```python
from build123d import *

# Parameters (mm, degrees)
SKETCH1_R           = 50
SKETCH1_W           = 15
SKETCH1_H           = 4
SKETCH1_W_2         = 4
SKETCH1_H_2         = 15
BOSS_EXTRUDE1_DEPTH = 5


with BuildPart() as part:
    # Sketch1 → Boss-Extrude1 (new body)
    with BuildSketch(Plane.XY):
        Circle(SKETCH1_R)
        with BuildLine():
            Line((-5, 14.142135624), (-5, 18.3))
            Line((-5, 18.3), (5, 18.3))
            Line((5, 18.3), (5, 14.142135624))
            ThreePointArc((5, 14.142135624), (0, -15), (-5, 14.142135624))
        make_face(mode=Mode.SUBTRACT)
        with Locations((-35, 0)):
            Rectangle(SKETCH1_W, SKETCH1_H, mode=Mode.SUBTRACT)
        Polygon((-38.499513267, 18.111804941), (-24.641320279, 12.371553455), (-26.172054009, 8.676035325), (-40.030246996, 14.41628681), align=None, mode=Mode.SUBTRACT)
        Polygon((-28.637824638, 31.466251763), (-18.03122292, 20.859650045), (-20.859650045, 18.03122292), (-31.466251763, 28.637824638), align=None, mode=Mode.SUBTRACT)
        Polygon((-14.41628681, 40.030246996), (-8.676035325, 26.172054009), (-12.371553455, 24.641320279), (-18.111804941, 38.499513267), align=None, mode=Mode.SUBTRACT)
        with Locations((0, 35)):
            Rectangle(SKETCH1_W_2, SKETCH1_H_2, mode=Mode.SUBTRACT)
        Polygon((18.111804941, 38.499513267), (12.371553455, 24.641320279), (8.676035325, 26.172054009), (14.41628681, 40.030246996), align=None, mode=Mode.SUBTRACT)
        Polygon((31.466251763, 28.637824638), (20.859650045, 18.03122292), (18.03122292, 20.859650045), (28.637824638, 31.466251763), align=None, mode=Mode.SUBTRACT)
        Polygon((40.030246996, 14.41628681), (26.172054009, 8.676035325), (24.641320279, 12.371553455), (38.499513267, 18.111804941), align=None, mode=Mode.SUBTRACT)
        with Locations((35, 0)):
            Rectangle(SKETCH1_W, SKETCH1_H, mode=Mode.SUBTRACT)
        Polygon((38.499513267, -18.111804941), (24.641320279, -12.371553455), (26.172054009, -8.676035325), (40.030246996, -14.41628681), align=None, mode=Mode.SUBTRACT)
        Polygon((28.637824638, -31.466251763), (18.03122292, -20.859650045), (20.859650045, -18.03122292), (31.466251763, -28.637824638), align=None, mode=Mode.SUBTRACT)
        Polygon((14.41628681, -40.030246996), (8.676035325, -26.172054009), (12.371553455, -24.641320279), (18.111804941, -38.499513267), align=None, mode=Mode.SUBTRACT)
        with Locations((0, -35)):
            Rectangle(SKETCH1_W_2, SKETCH1_H_2, mode=Mode.SUBTRACT)
        Polygon((-18.111804941, -38.499513267), (-12.371553455, -24.641320279), (-8.676035325, -26.172054009), (-14.41628681, -40.030246996), align=None, mode=Mode.SUBTRACT)
        Polygon((-31.466251763, -28.637824638), (-20.859650045, -18.03122292), (-18.03122292, -20.859650045), (-28.637824638, -31.466251763), align=None, mode=Mode.SUBTRACT)
        Polygon((-40.030246996, -14.41628681), (-26.172054009, -8.676035325), (-24.641320279, -12.371553455), (-38.499513267, -18.111804941), align=None, mode=Mode.SUBTRACT)
    extrude(amount=BOSS_EXTRUDE1_DEPTH)


solid = part.part
```
The listing builds one solid part. Answer for the finished solid, in the listing's coordinates (mm). Give positions to 0.01 mm unless a question says otherwise; leave off trailing zeros. Order: outer loops, then holes, each group sorted by start corner. A loop starts at its lowest first (then second) coordinate and runs counter-clockwise, first axis right, second up. Notation, with made-up numbers: (-25, 37) -> (-13, 37) arc R23 cw to (-13, 56) -> close; hole circle Ø7 at (6, 17). An arc over 180 degrees is marked (long way). Write each question's results on one line, items separated by ' | '.
Q1. The part is cut by section D-D, the plane z = 2.5. State how many separate pieces and enclosed holes the cut face has, and give its area (3 significant figures).
Checked values:
separate pieces: 1 | enclosed holes: 17 | area: 6,150 mm^2
Q2. The part is cut by section B-B, the plane x = 0. Give the vertices of the cut face in (y, z), and give its area (4 significant figures).
Checked values:
outline: (-50, 0) -> (-42.5, 0) -> (-42.5, 5) -> (-50, 5) -> close; (-27.5, 0) -> (-15, 0) -> (-15, 5) -> (-27.5, 5) -> close; (18.3, 0) -> (27.5, 0) -> (27.5, 5) -> (18.3, 5) -> close; (42.5, 0) -> (50, 0) -> (50, 5) -> (42.5, 5) -> close | area: 183.5 mm^2
Q3. Each of these flat-tipped pins is pushed along its axis until it touches: P1, Ø2.5, axis at x = 32, z = 3, coming from the -Y side; P2, Ø2.5, axis at y = 37, z = 3.5, coming from the +X side; P3, Ø3, axis at y = -0.5, z = 3, coming from the +X side; P4, Ø3, axis at x = 1, z = 3, coming from the -Y side. Where does it stop, or does it pass through?
Checked values:
P1: stops at y = -39.43 | P2: stops at x = 34.96 | P3: stops at x = 50 | P4: stops at y = -50
Q4. The part is cut by section A-A, the plane y = 0. Give the vertices of the cut face in (x, z), and give its area (3 significant figures).
Checked values:
outline: (-50, 0) -> (-42.5, 0) -> (-42.5, 5) -> (-50, 5) -> close; (-27.5, 0) -> (-15, 0) -> (-15, 5) -> (-27.5, 5) -> close; (15, 0) -> (27.5, 0) -> (27.5, 5) -> (15, 5) -> close; (42.5, 0) -> (50, 0) -> (50, 5) -> (42.5, 5) -> close | area: 200 mm^2
Q5. Determine the mould class of faces 1 (the face through (10, 12, 0)), 2 (the face through (-33.004, 11.506, 2.465)), 3 (the face through (47.69, 15.02, 2.46)) for opening direction Y: pulls with the +Y half, pulls with the -Y half, needs draft (parallel to the pull), parting line crosses it, or undercut.
Checked values:
face 1: needs draft | face 2: undercut | face 3: parting line crosses it
Q6. The part is cut by section C-C, the plane x = 22.5. Give the vertices of the cut face in (y, z).
Checked values:
outline: (-44.65, 0) -> (-25.33, 0) -> (-25.33, 5) -> (-44.65, 5) -> close; (-19.67, 0) -> (19.67, 0) -> (19.67, 5) -> (-19.67, 5) -> close; (25.33, 0) -> (44.65, 0) -> (44.65, 5) -> (25.33, 5) -> close
Q7. Straight lines are drawn through the part: probe 1 along Y at (x, z) = (0, 2.2); probe 2 along Y at (x, z) = (-35.5, 1.1); probe 3 along X at (y, z) = (-1, 3.15). For each, find the intervals that lie inside material, in ascending order. Write a range as from..to.
Checked values:
probe 1: y = -50..-42.5, -27.5..-15, 18.3..27.5, 42.5..50 | probe 2: y = -35.21..-16.87, -12.54..-2, 2..12.54, 16.87..35.21 | probe 3: x = -49.99..-42.5, -27.5..-14.97, 14.97..27.5, 42.5..49.99
